Check sheet for the drawn part. Datum: minimum x, y, z corner. Units: mm. A direction names the side the tool comes from. Round coordinates to 2 decimals unless told otherwise and drop trailing zeros. Order: outer loops, then holes, each group sorted by start corner. A loop starts at its lowest first (then second) coordinate and runs counter-clockwise, first axis right, second up.
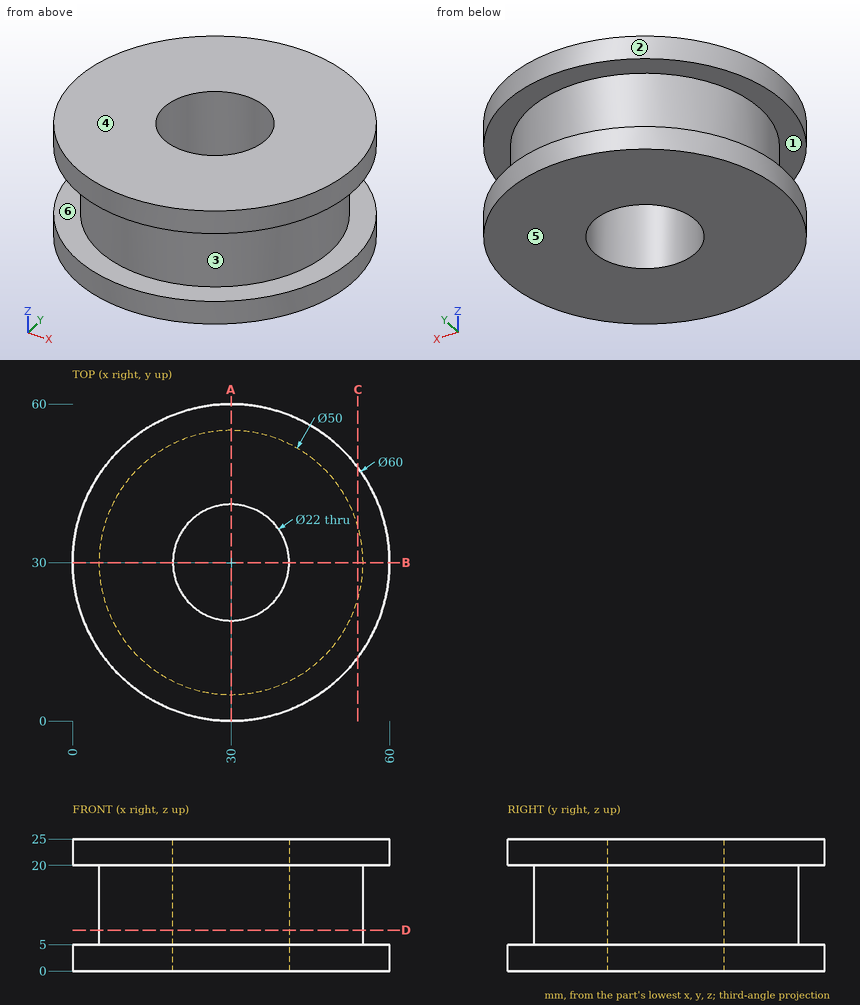
(1) Set-up check for the marked faces 5 and 6: record each of +Z, -Z, +X, -X, +Y, -Y from which the full face is reachable in a straight line by a thin tool's end or side.
Returned:
face 5: -Z, +X, -X, +Y, -Y
face 6: none
(2) Sectioned sample at A-A, the plane x = 30. Record the cut outline in (y, z).
Returned:
outline: (0, 0) - (19, 0) - (19, 25) - (0, 25) - (0, 20) - (5, 20) - (5, 5) - (0, 5) - close; (41, 0) - (60, 0) - (60, 5) - (55, 5) - (55, 20) - (60, 20) - (60, 25) - (41, 25) - close
(3) Sectioned sample at C-C, the plane x = 54. Record the cut outline in (y, z).
Returned:
outline: (12, 0) - (48, 0) - (48, 5) - (37, 5) - (37, 20) - (48, 20) - (48, 25) - (12, 25) - (12, 20) - (23, 20) - (23, 5) - (12, 5) - close
(4) Draft check along Z on the marked faces 1, 2, 3 and 4. Enter one of: released by +Z, released by -Z, zero draft, split by the parting line, or undercut.
Returned:
face 1: undercut
face 2: zero draft
face 3: undercut
face 4: released by +Z
(5) Material ranges on line 1 (Z direction, x = 54, y = 22.5); line 2 (Y direction, x = 30, z = 8.75); line 3 (X direction, y = 21, z = 8.25), recorded low to high.
Returned:
line 1: z = 0 to 5, 20 to 25
line 2: y = 5 to 19, 41 to 55
line 3: x = 6.68 to 23.68, 36.32 to 53.32
(6) Sectioned sample at D-D, the plane z = 7.75. Record the cut outline in (x, y).
Returned:
outline: circle Ø50 at (30, 30); hole circle Ø22 at (30, 30)
(7) Depth check by flat-ended pin: P1, Ø4, axis at x = 44, y = 50.5, coming from the -Z side; P2, Ø12, axis at x = 45.5, z = 8, coming from the -Y side (3 decimals); P3, Ø10, axis at x = 26, z = 3.5, coming from the +Y side; P4, Ø1.5, axis at y = 40.5, z = 11, coming from the +X side. Enter the tip coordinate at first touch or a pass-through.
Returned:
P1: stops at z = 0
P2: stops at y = 1.825
P3: stops at y = 60
P4: stops at x = 53.02
